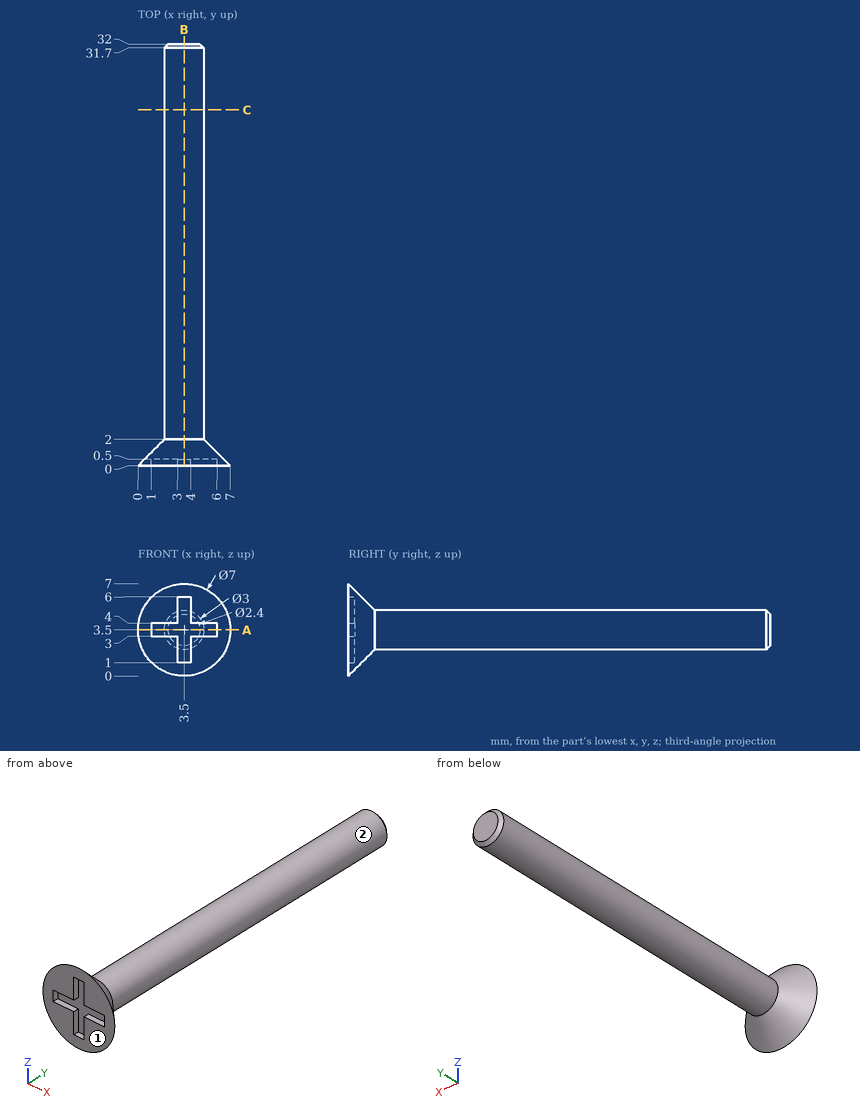
Here's the drawing with two shaded views (mm, measured from the low corner). I have some questions. A direction names the side the tool comes from. Round coordinates to 2 decimals unless told otherwise and drop trailing zeros. Write each loop counter-clockwise with the first axis right and the second up, starting at its lowest first coordinate (ties: lowest second). Pieces come first, ordered by that corner, then holes.
(1) For pin 1 (1.5 mm diameter, centred on x = 1.5, y = 4, fed in from +Z); pin 2 (0.6 mm diameter, centred on x = 5, y = 0.5, fed in from -Z); pin 3 (0.6 mm diameter, centred on x = 5, y = 0.5, fed in from +Z); pin 4 (1.5 mm diameter, centred on x = 3.5, z = 4, fed in from -Y), each with a flat end and sliding along its axis, tell me the tip position at first contact or that it passes through.
Findings below:
pin 1: stops at z = 4.33
pin 2: stops at z = 0.53
pin 3: stops at z = 6.47
pin 4: stops at y = 0
(2) If I drill on probe 1 along Y at (x, z) = (5.5, 1.5); probe 2 along X at (y, z) = (4, 2.5); probe 3 along Y at (x, z) = (2, 5.5), over which ranges is the centre line in solid material (lowest first)?
Findings below:
probe 1: y = 0 to 0.67
probe 2: x = 2.38 to 4.62
probe 3: y = 0 to 1
(3) Suppose I cut it at C-C on y = 27. Write out the boundary of the cut face in (x, z).
Findings below:
outline: circle Ø3 at (3.5, 3.5)
(4) Suppose I cut it at A-A on z = 3.5. Write out the boundary of the cut face in (x, y).
Findings below:
outline: (0, 0) - (1, 0) - (1, 0.5) - (6, 0.5) - (6, 0) - (7, 0) - (5, 2) - (5, 31.7) - (4.7, 32) - (2.3, 32) - (2, 31.7) - (2, 2) - close
(5) Suppose I cut it at B-B on x = 3.5. Write out the boundary of the cut face in (y, z), and give its area (3 significant figures).
Findings below:
outline: (0, 0) - (2, 2) - (31.7, 2) - (32, 2.3) - (32, 4.7) - (31.7, 5) - (2, 5) - (0, 7) - (0, 6) - (0.5, 6) - (0.5, 1) - (0, 1) - close
area: 97.4 mm2
(6) Which directions (+Z, -Z, +X, -X, +Y, -Y) give clear straight access to the entire face, cutting with the end or side of a thin tool? Please do the marked faces 1 and 2.
Findings below:
face 1: +Z, -Z, +X, -X, -Y
face 2: +Y
